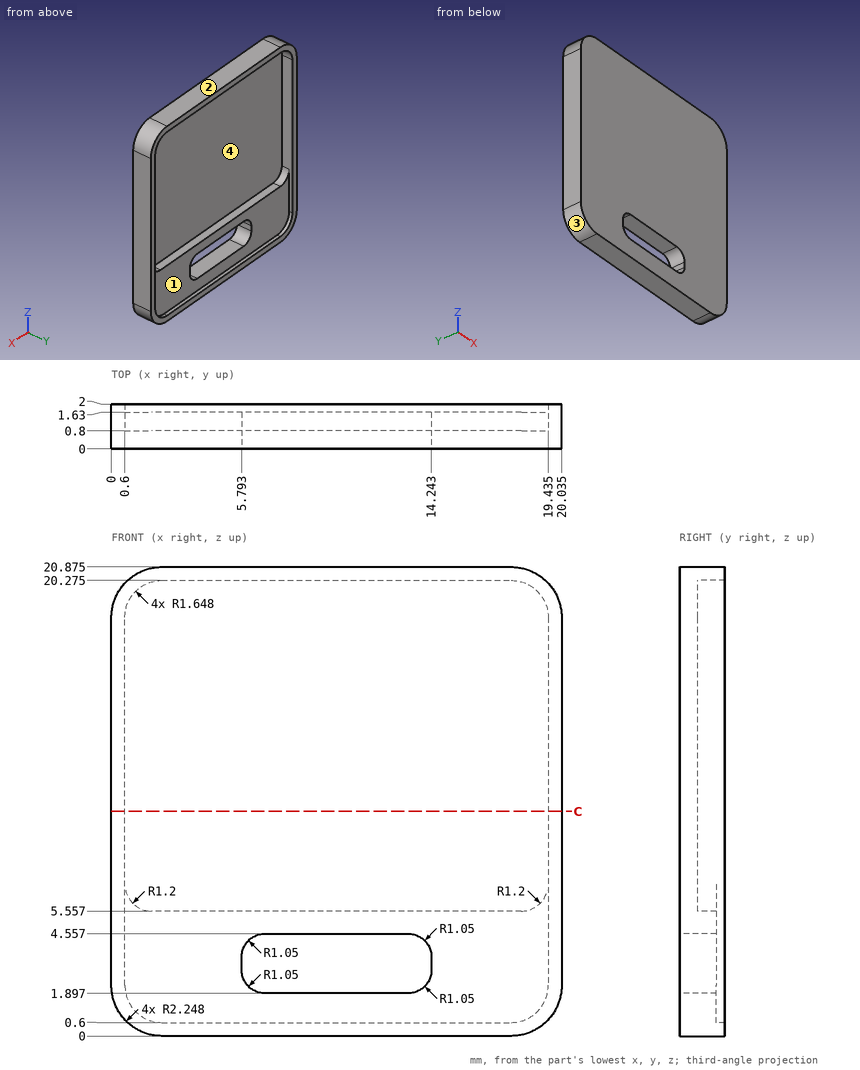
Design review of the part shown in the three views and the two pictorial views. Dimensions are in mm from the part's minimum x, y and z. Give positions to 0.01 mm unless a question says otherwise; leave off trailing zeros. Write each loop counter-clockwise with the first axis right and the second up, starting at its lowest first coordinate (ties: lowest second). Pieces come first, ordered by that corner, then holes. Notation, with made-up numbers: M -9.5,19 L -3.5,19 A8 ccw -3.5,34 Z; hole C 78,78 d6. An arc over 180 degrees is marked long. Return JSON: item names as keys, results as strings. Group by question number.
Item 1: The part is to be moulded in two halves that separate along X. For the marked faces 1, 2, 3 and 4, say which applies: pulls with the +X half, pulls with the -X half, needs draft (parallel to the pull), parting line crosses it, or undercut.
Item 2: Wall thickness on line 1 along Z through (x, y) = (7.5, 1.25) (1 decimal); line 2 along Z through (x, y) = (4.75, 1.4) (1 decimal); line 3 along X through (y, z) = (1.9, 10.5) (1 decimal): over which ranges is each line inside the solid? List them lowest first.
Item 3: Take a section at C-C (z = 10). Give the boundary of the cut face in (x, y) (1 decimal).
Item 4: Clearance check with a flat-ended pin moving along its axis: pin 1 Ø1.5 at (x, z) = (15, 14) entering from +Y. State where the tip first meets the part, or that it passes through.
Return value:
{
 "1": {"face 1": "undercut", "face 2": "needs draft", "face 3": "pulls with the -X half", "face 4": "undercut"},
 "2": {"line 1": "z = 0 to 1.9, 4.6 to 5.6, 20.3 to 20.9", "line 2": "z = 0 to 5.6, 20.3 to 20.9", "line 3": "x = 0 to 0.6, 19.4 to 20"},
 "3": {"outline": "M 0,0 L 20,0 L 20,2 L 19.4,2 L 19.4,0.8 L 0.6,0.8 L 0.6,2 L 0,2 Z"},
 "4": {"pin 1": "stops at y = 0.8"}
}
